Input: part model. Units: mm. Frame: model coordinates. Round coordinates to 2 decimals unless told otherwise and drop trailing zeros. Loops run counter-clockwise (first coordinate to the right, second up) from the corner with the lowest first, then second, coordinate; pieces in that order, holes last. Notation, with made-up numbers: (3.5, 54.5) -> (27.5, 54.5) arc R22 cw to (27.5, 61.5) -> close; hole circle Ø1 at (58.5, 37.5). An arc over 180 degrees is marked (long way). Answer as a JSON object with one key per item and string values.
Autodesk Inventor part; units mm, degrees
ref_plane "Work Plane1" through (0, 0, 0) normal (0, 0, 1) x (1, 0, 0)
ref_plane "YZ Plane" through (0, 0, 0) normal (1, 0, 0) x (0, 1, 0)
ref_plane "XZ Plane" through (0, 0, 0) normal (0, 1, 0) x (-1, 0, 0)
ref_plane "Work Plane1" through (0, 0, 0) normal (0, 0, 1) x (1, 0, 0)
sketch "Sketch1" plane through (0, 0, 0) normal (0, 0, 1) x (1, 0, 0)
  line L0 (-560, 55) -> (-11.1724, 304.4671) construction
  line L1 (-10.3448, 302.6464) -> (-559.1724, 53.1793)
  line L2 (-559.1724, 53.1793) -> (-560, 55)
  line L3 (-10, 600) -> (0, 600) construction
  line L4 (0, 600) -> (0, 0) construction
  line L5 (0, 0) -> (-10, 0) construction
  line L6 (-10, 0) -> (-10, 600) construction
  line L7 (-10, 17.7053) -> (-559.1724, 17.7053)
  line L8 (-559.1724, 53.1793) -> (-559.1724, 17.7053)
  line L9 (-559.1724, 17.7053) -> (-10, 17.7053)
  line L10 (-10, 17.7053) -> (-10, 0)
  line L11 (-10, 0) -> (-559.1724, 0)
  line L12 (-559.1724, 0) -> (-559.1724, 17.7053)
  line L13 (-10, 302.6464) -> (-10.3448, 302.6464)
  line L14 (-10, 17.7053) -> (-10, 302.6464)
  point P0 (-10, 202.6464)
extrude "Extrusion5" add sketch "Sketch1" along normal mid plane 10
sketch "Sketch2" plane through (0, 0, 5) normal (0, 0, 1) x (1, 0, 0)
  line L0 (-559.1724, 53.1793) -> (-559.1724, 0)
  line L1 (-559.1724, 0) -> (-555.1724, 0)
  line L2 (-555.1724, 0) -> (-555.1724, 80)
  line L3 (-555.1724, 80) -> (-559.1724, 80)
  line L4 (-559.1724, 80) -> (-559.1724, 0)
  point P0 (0, 0)
  dimension "d10" = 4
  dimension "d11" = 80
extrude "Extrusion6" cut sketch "Sketch2" against normal through all
properties part number "verticalff1" material "Wood (Birch)"
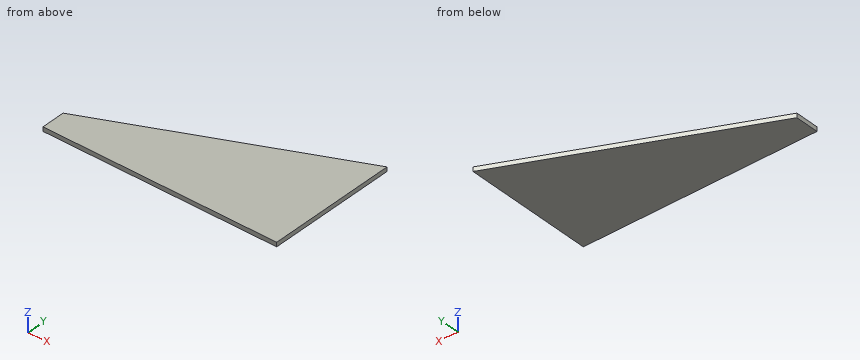
1) Section A-A, the plane z = 2. Output: boundary loops of the cut face in (x, y).
Output:
{"outline": "(-555.17, 0) -> (-10, 0) -> (-10, 302.65) -> (-10.34, 302.65) -> (-555.17, 55) -> close"}
2) Section C-C, the plane y = 61. Output: boundary loops of the cut face in (x, z), plus the area to 3 significant figures.
Output:
{"outline": "(-541.97, -5) -> (-10, -5) -> (-10, 5) -> (-541.97, 5) -> close", "area": "5,320 mm^2"}
3) Section B-B, the plane x = -150. Output: boundary loops of the cut face in (y, z).
Output:
{"outline": "(0, -5) -> (239.17, -5) -> (239.17, 5) -> (0, 5) -> close"}
4) Ray query, probe 1 along X at (y, z) = (220.5, -1.25); probe 2 along Y at (x, z) = (-518, -1.5); probe 3 along X at (y, z) = (107, -4). Return the intervals inside material, ascending.
Output:
{"probe 1": "x = -191.07 to -10", "probe 2": "y = 0 to 71.89", "probe 3": "x = -440.77 to -10"}
5) Contact query for a flat-ended pin moving along its axis: P1, Ø5, axis at x = -355.5, z = 2, coming from the +Y side. Output: stop coordinate, or through.
Output:
{"P1": "stops at y = 146.89"}
